Model file for the job. Use its own axes, mm. Face numbers are marked on the shaded views. A direction names the side the tool comes from. Give positions to 0.01 mm unless a question says otherwise; leave off trailing zeros. Order: outer loops, then holes, each group sorted by start corner. A loop starts at its lowest first (then second) coordinate and runs counter-clockwise, first axis right, second up. Notation, with made-up numbers: (19, 44) -> (37, 44) arc R28 cw to (37, 66) -> close; hole circle Ø7 at (-33, 14). An arc over 180 degrees is marked (long way). Use CSV: the item, a comma, the result in double quotes. Start each with the question number.
1. Wall check: line 1 (X direction, y = -0.25, z = 7.5); line 2 (Z direction, x = 23, y = 1.5); line 3 (Y direction, x = 0, z = 11.5). Give the ranges that are in metal, low to high. Write a range as from..to.
2. 3-axis set-ups, long thin cutter, end or side, ignore diameter. For the marked faces 1, 2 and 3: which of +Z, -Z, +X, -X, +Y, -Y reach the whole face in a straight line?
3. Cut at B-B on x = 23. List the corners of the cut face in (y, z).
4. Drop flat-ended pins along their axis: pin 1 (8 mm diameter, centred on y = 18, z = 7, fed in from -X); pin 2 (9 mm diameter, centred on x = 0, y = 15, fed in from +Z); pin 3 (4 mm diameter, centred on x = 23, z = 10, fed in from +Y); pin 4 (1 mm diameter, centred on y = 21.5, z = 9, fed in from +X). Give the stop position or say it passes through.
5. Pull direction Z, two halves, no side cores. Call the marked faces 4, 5 and 6: released by +Z, released by -Z, zero draft, split by the parting line, or undercut.
6. Cut at A-A on z = 4. List the corners of the cut face in (x, y).
7. Cut at C-C on y = 15. List the corners of the cut face in (x, z).
8. Cut at D-D on z = 7.5. List the corners of the cut face in (x, y), then the cut area to 3 significant figures.
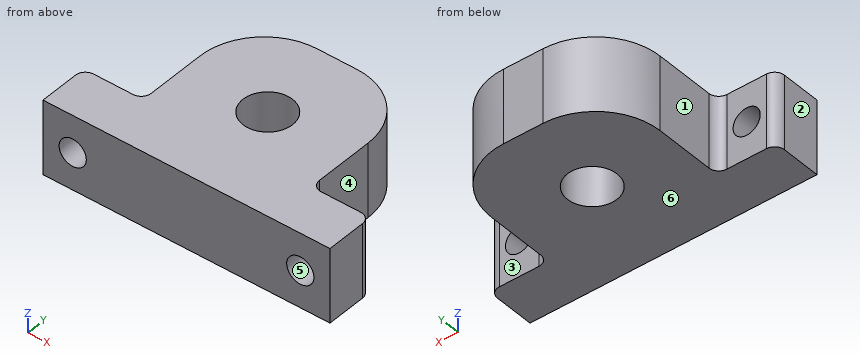
```python
from build123d import *

# Parameters (mm, degrees)
SKETCH_1_W          = 58
SKETCH_1_H          = 10
SKETCH_1_W_2        = 34
SKETCH_1_H_2        = 27
SKETCH_1_R          = 5
EXTRUDE_1_DEPTH     = 15
SKETCH_2_R          = 2.75
CUT_EXTRUDE_1_DEPTH = 15
FILLET_2_R          = 13
FILLET_3_R          = 2


with BuildPart() as part:
    # 草图1 → 凸台-拉伸1 (new body)
    with BuildSketch(Plane.XY):
        Rectangle(SKETCH_1_W, SKETCH_1_H)
        with Locations((0, 18.5)):
            Rectangle(SKETCH_1_W_2, SKETCH_1_H_2)
        with Locations((0, 15)):
            Circle(SKETCH_1_R, mode=Mode.SUBTRACT)
    extrude(amount=EXTRUDE_1_DEPTH)

    # 草图2 → 切除-拉伸1 (cut)
    with BuildSketch(Plane(origin=(0, 5, 0), x_dir=(1, 0, 0), z_dir=(0, 1, 0))):
        with Locations((-23, -7.5)):
            Circle(SKETCH_2_R)
        with Locations((23, -7.5)):
            Circle(SKETCH_2_R)
    extrude(amount=-CUT_EXTRUDE_1_DEPTH, mode=Mode.SUBTRACT)

    # 圆角2
    fillet_2_edges = [part.edges().sort_by_distance(p)[0] for p in [
        (-17, 32, 7.5),
        (17, 32, 7.5),
    ]]
    fillet(fillet_2_edges, radius=FILLET_2_R)

    # 圆角3
    fillet_3_edges = [part.edges().sort_by_distance(p)[0] for p in [
        (-29, 5, 7.5),
        (-17, 5, 7.5),
        (17, 5, 7.5),
        (29, 5, 7.5),
    ]]
    fillet(fillet_3_edges, radius=FILLET_3_R)


solid = part.part
```
Verdict:
1,line 1,"-29..-25.75, -20.25..20.25, 25.75..29"
1,line 2,"0..4.75, 10.25..15"
1,line 3,"-5..10, 20..32"
2,face 1,"+Z, -Z, -X, +Y"
2,face 2,"+Z, -Z, -X, +Y, -Y"
2,face 3,"+Z, -Z, +X, +Y"
3,outline,"(-5, 0) -> (5, 0) -> (5, 4.75) -> (-5, 4.75) -> close; (-5, 10.25) -> (5, 10.25) -> (5, 15) -> (-5, 15) -> close"
4,pin 1,"x = -17"
4,pin 2,"through"
4,pin 3,"y = 5"
4,pin 4,"x = 16.85"
5,face 4,"zero draft"
5,face 5,"undercut"
5,face 6,"released by -Z"
6,outline,"(-29, -5) -> (29, -5) -> (29, 3) arc R2 ccw to (27, 5) -> (19, 5) arc R2 cw to (17, 7) -> (17, 19) arc R13 ccw to (4, 32) -> (-4, 32) arc R13 ccw to (-17, 19) -> (-17, 7) arc R2 cw to (-19, 5) -> (-27, 5) arc R2 ccw to (-29, 3) -> close; hole circle Ø10 at (0, 15)"
7,outline,"(-17, 0) -> (-5, 0) -> (-5, 15) -> (-17, 15) -> close; (5, 0) -> (17, 0) -> (17, 15) -> (5, 15) -> close"
8,outline,"(-29, -5) -> (-25.75, -5) -> (-25.75, 5) -> (-27, 5) arc R2 ccw to (-29, 3) -> close; (-20.25, -5) -> (20.25, -5) -> (20.25, 5) -> (19, 5) arc R2 cw to (17, 7) -> (17, 19) arc R13 ccw to (4, 32) -> (-4, 32) arc R13 ccw to (-17, 19) -> (-17, 7) arc R2 cw to (-19, 5) -> (-20.25, 5) -> close; (25.75, -5) -> (29, -5) -> (29, 3) arc R2 ccw to (27, 5) -> (25.75, 5) -> close; hole circle Ø10 at (0, 15)"
8,area,"1,240 mm^2"
